from build123d import *

# Parameters (mm, degrees)
SKETCH1_W                       = 20.32
SKETCH1_H                       = 50.8
BOSS_EXTRUDE1_DEPTH             = 1.6002
CHAMFER1_SIZE                   = 5.08
F_3_CLEARANCE_HOLE1_D           = 2.794
F_3_CLEARANCE_HOLE1_DEPTH       = 11.43
F_3_CLEARANCE_HOLE1_CSINK_D     = 4.064
F_3_CLEARANCE_HOLE1_CSINK_ANGLE = 90
F_3_CLEARANCE_HOLE1_TIP         = 0.839402285
F_8_CLEARANCE_HOLE1_D           = 4.3053


with BuildPart() as part:
    # Sketch1 → Boss-Extrude1 (new body)
    with BuildSketch(Plane.XY):
        Rectangle(SKETCH1_W, SKETCH1_H)
    extrude(amount=BOSS_EXTRUDE1_DEPTH)

    # Chamfer1
    chamfer1_edges = [part.edges().sort_by_distance(p)[0] for p in [
        (10.16, -25.4, 0.8001),
    ]]
    chamfer(chamfer1_edges, length=CHAMFER1_SIZE)

    # #3 Clearance Hole1
    with Locations(Plane(origin=(-1.5494, -7.62, 1.6002), x_dir=(1, 0, 0), z_dir=(0, 0, 1))):
        with Locations((0, 0), (0, 25)):
            CounterSinkHole(F_3_CLEARANCE_HOLE1_D / 2, F_3_CLEARANCE_HOLE1_CSINK_D / 2, depth=F_3_CLEARANCE_HOLE1_DEPTH, counter_sink_angle=F_3_CLEARANCE_HOLE1_CSINK_ANGLE)
            with Locations((0, 0, -(F_3_CLEARANCE_HOLE1_DEPTH + F_3_CLEARANCE_HOLE1_TIP / 2))):  # 118° drill point
                Cone(0, F_3_CLEARANCE_HOLE1_D / 2, F_3_CLEARANCE_HOLE1_TIP, mode=Mode.SUBTRACT)

    # #8 Clearance Hole1 (through all)
    with Locations(Plane(origin=(1.143, -17.78, 1.6002), x_dir=(1, 0, 0), z_dir=(0, 0, 1))):
        with Locations((0, 0)):
            Hole(F_8_CLEARANCE_HOLE1_D / 2)


solid = part.part
Model file for the job. Use its own axes, mm. Round coordinates to 2 decimals unless told otherwise and drop trailing zeros. Order: outer loops, then holes, each group sorted by start corner. A loop starts at its lowest first (then second) coordinate and runs counter-clockwise, first axis right, second up. Notation, with made-up numbers: M 46.5,46.25 L 96.5,46.25 A17 cw 96.5,56.25 Z; hole C 43.25,20 d3. An arc over 180 degrees is marked long. Write each question's results on one line, items separated by ' | '. Start each with the question number.
(1) Saw through at D-D, the plane z = 1.35. Give the cut face in (x, y), then the cut area to 3 significant figures.
(2) Probe probe 1 along Y at (x, z) = (-1.25, 0.7); probe 2 along Y at (x, z) = (-2, 0.25); probe 3 along X at (y, z) = (-7.62, 0.2). List the from-to ranges inside material, lowest first. Write a range as from..to.
(3) Drop a flat-ended pin along its axis: pin 1 (6 mm diameter, centred on x = -1, y = 10.5, fed in from -Z). Give the stop position or say it passes through.
(4) Two-plate mould, pull along X, no slides. Class faces 1 (the face through (-1.247, -8.984, 0.476)), 2 (the face through (0, 25.4, 1)), 3 (the face through (10.16, 2, 1)): pulls with the +X half, pulls with the -X half, needs draft (parallel to the pull), parting line crosses it, or undercut.
(5) Saw through at B-B, the plane x = 2.5. Give the cut face in (y, z).
(6) Saw through at C-C, the plane y = -7.62. Give the cut face in (x, z), then the cut area to 3 significant figures.
(7) Saw through at A-A, the plane y = -17.78. Give the cut face in (x, z).
Established:
1) outline: M -10.16,-25.4 L 5.08,-25.4 L 10.16,-20.32 L 10.16,25.4 L -10.16,25.4 Z; hole C -1.55,-7.62 d3.56; hole C -1.55,17.38 d3.56; hole C 1.14,-17.78 d4.31 | area: 985 mm^2
2) probe 1: y = -25.4..-8.98, -6.26..16.02, 18.74..25.4 | probe 2: y = -25.4..-8.94, -6.3..16.06, 18.7..25.4 | probe 3: x = -10.16..-2.95, -0.15..10.16
3) pin 1: stops at z = 0
4) face 1: undercut | face 2: needs draft | face 3: pulls with the +X half
5) outline: M -25.4,0 L -19.45,0 L -19.45,1.6 L -25.4,1.6 Z; M -16.11,0 L 25.4,0 L 25.4,1.6 L -16.11,1.6 Z
6) outline: M -10.16,0 L -2.95,0 L -2.95,0.97 L -3.58,1.6 L -10.16,1.6 Z; M -0.15,0 L 10.16,0 L 10.16,1.6 L 0.48,1.6 L -0.15,0.97 Z | area: 27.6 mm^2
7) outline: M -10.16,0 L -1.01,0 L -1.01,1.6 L -10.16,1.6 Z; M 3.3,0 L 10.16,0 L 10.16,1.6 L 3.3,1.6 Z
